Work out the finished part from the listing and answer in its coordinate system (mm). A direction names the side the tool comes from. Give positions to 0.01 mm unless a question says otherwise; leave off trailing zeros. Order: outer loops, then holes, each group sorted by start corner. A loop starts at its lowest first (then second) coordinate and runs counter-clockwise, first axis right, second up.
```python
from build123d import *

# Parameters (mm, degrees)
SKETCH1_W           = 200
SKETCH1_H           = 200
BOSS_EXTRUDE1_DEPTH = 200
SKETCH3_W           = 200
SKETCH3_H           = 12.5
BOSS_EXTRUDE2_DEPTH = 20
SKETCH4_W           = 220
SKETCH4_H           = 12.5
BOSS_EXTRUDE3_DEPTH = 20
SKETCH5_W           = 220
SKETCH5_H           = 12.5
BOSS_EXTRUDE4_DEPTH = 20
SKETCH6_W           = 240
SKETCH6_H           = 12.5
BOSS_EXTRUDE5_DEPTH = 20
FILLET1_R           = 50
FILLET2_R           = 5
SHELL1_T            = -4


with BuildPart() as part:
    # Sketch1 → Boss-Extrude1 (new body)
    with BuildSketch(Plane(origin=(0, 0, 0), x_dir=(1, 0, 0), z_dir=(0, 1, 0))):
        with Locations((100, 100)):
            Rectangle(SKETCH1_W, SKETCH1_H)
    extrude(amount=BOSS_EXTRUDE1_DEPTH)

    # Sketch3 → Boss-Extrude2 (add)
    with BuildSketch(Plane.XY):
        with Locations((100, 6.25)):
            Rectangle(SKETCH3_W, SKETCH3_H)
    extrude(amount=BOSS_EXTRUDE2_DEPTH)

    # Sketch4 → Boss-Extrude3 (add)
    with BuildSketch(Plane(origin=(200, 0, 0), x_dir=(0, 0, -1), z_dir=(1, 0, 0))):
        with Locations((90, 6.25)):
            Rectangle(SKETCH4_W, SKETCH4_H)
    extrude(amount=BOSS_EXTRUDE3_DEPTH)

    # Sketch5 → Boss-Extrude4 (add)
    with BuildSketch(Plane(origin=(0, 0, -200), x_dir=(-1, 0, 0), z_dir=(0, 0, -1))):
        with Locations((-110, 6.25)):
            Rectangle(SKETCH5_W, SKETCH5_H)
    extrude(amount=BOSS_EXTRUDE4_DEPTH)

    # Sketch6 → Boss-Extrude5 (add)
    with BuildSketch(Plane.ZY):
        with Locations((-100, 6.25)):
            Rectangle(SKETCH6_W, SKETCH6_H)
    extrude(amount=BOSS_EXTRUDE5_DEPTH)

    # Fillet1
    fillet1_edges = [part.edges().sort_by_distance(p)[0] for p in [
        (220, 6.25, 20),
        (220, 6.25, -220),
        (-20, 6.25, -220),
        (-20, 6.25, 20),
    ]]
    fillet(fillet1_edges, radius=FILLET1_R)

    # Fillet2
    fillet2_edges = [part.edges().sort_by_distance(p)[0] for p in [
        (200, 200, -100),
        (100, 200, -200),
        (0, 200, -100),
        (100, 200, 0),
        (0, 106.25, -200),
        (200, 106.25, -200),
        (200, 106.25, 0),
        (0, 106.25, 0),
    ]]
    fillet(fillet2_edges, radius=FILLET2_R)

    # Shell1
    shell1_openings = [part.faces().sort_by_distance(p)[0] for p in [
        (100, 0, -100),
    ]]
    offset(amount=SHELL1_T, openings=shell1_openings, kind=Kind.INTERSECTION)


solid = part.part
```
1. Straight lines are drawn through the part: probe 1 along Z at (x, y) = (34, 53); probe 2 along X at (y, z) = (102.5, -93); probe 3 along Y at (x, z) = (202, -172). For each, find the intervals that lie inside material, in ascending order.
Findings below:
probe 1: z = -200 to -196, -4 to 0
probe 2: x = 0 to 4, 196 to 200
probe 3: y = 8.5 to 12.5
2. The mould has two halves that part along X. Classify faces 1 (the face through (204.964, 6.338, 5.742)), 2 (the face through (202.17, 4.31, 2.88)), 3 (the face through (196, 100, -101)), 4 (the face through (99, 102, 0)): pulls with the +X half, pulls with the -X half, needs draft (parallel to the pull), parting line crosses it, or undercut.
Findings below:
face 1: pulls with the +X half
face 2: undercut
face 3: undercut
face 4: needs draft
3. The part is cut by section A-A (y = 133). Write down the section's boundary in (x, z), then the cut area to 3 significant figures.
Findings below:
outline: (0, -195) arc R5 ccw to (5, -200) - (195, -200) arc R5 ccw to (200, -195) - (200, -5) arc R5 ccw to (195, 0) - (5, 0) arc R5 ccw to (0, -5) - close; hole (4, -195) arc R1 ccw to (5, -196) - (195, -196) arc R1 ccw to (196, -195) - (196, -5) arc R1 ccw to (195, -4) - (5, -4) arc R1 ccw to (4, -5) - close
area: 3,120 mm2
4. The part is cut by section B-B (x = 156). Write down the section's boundary in (y, z), then the cut area to 3 significant figures.
Findings below:
outline: (0, -220) - (12.5, -220) - (12.5, -200) - (195, -200) arc R5 ccw to (200, -195) - (200, -5) arc R5 ccw to (195, 0) - (12.5, 0) - (12.5, 20) - (0, 20) - (0, 16) - (8.5, 16) - (8.5, -4) - (195, -4) arc R1 cw to (196, -5) - (196, -195) arc R1 cw to (195, -196) - (8.5, -196) - (8.5, -216) - (0, -216) - close
area: 2,520 mm2
5. The part is cut by section D-D (x = -4). Write down the section's boundary in (y, z).
Findings below:
outline: (0, -206.66) - (12.5, -206.66) - (12.5, 6.66) - (0, 6.66) - (0, 0.98) - (8.5, 0.98) - (8.5, -200.98) - (0, -200.98) - close
6. Which of the six approach directions +Z, -Z, +X, -X, +Y, -Y give full straight-line access (tool end or side, diameter ignored) to faces 5 (the face through (99, 102, -200)), 6 (the face through (101, 4, -216)), 7 (the face through (-6, 12.5, -101)), 8 (the face through (-20, 6, -101)), 9 (the face through (200, 102, -101))?
Findings below:
face 5: -Z, +X, -X, +Y
face 6: -Y
face 7: +Y
face 8: +Z, -Z, -X, +Y, -Y
face 9: +Z, -Z, +X, +Y
7. Given P1, Ø12, axis at y = 173, z = -114, coming from the +X side; P2, Ø2, axis at x = 39.5, z = -159.5, coming from the -Y side; P3, Ø1, axis at y = 83.5, z = -23, coming from the -X side, each flat-ended and moving along its own axis, determine where each tip first touches the part or whether it passes through.
Findings below:
P1: stops at x = 200
P2: stops at y = 196
P3: stops at x = 0
8. The part is cut by section C-C (z = -115). Write down the section's boundary in (x, y), then the cut area to 3 significant figures.
Findings below:
outline: (-20, 0) - (-16, 0) - (-16, 8.5) - (4, 8.5) - (4, 195) arc R1 cw to (5, 196) - (195, 196) arc R1 cw to (196, 195) - (196, 8.5) - (216, 8.5) - (216, 0) - (220, 0) - (220, 12.5) - (200, 12.5) - (200, 195) arc R5 ccw to (195, 200) - (5, 200) arc R5 ccw to (0, 195) - (0, 12.5) - (-20, 12.5) - close
area: 2,520 mm2
